Can you work these out from the model? Positions are in its coordinate system, mm. A direction names the side the tool comes from. Coordinates: 2 decimals unless noted, no trailing zeros. Order: outer loops, then holes, each group sorted by start corner. A loop starts at its lowest first (then second) coordinate and runs counter-clockwise, first axis right, second up.
Solid Edge part; units mm, degrees
sketch "Sketch1" plane through (0, 0, 0) normal (0, 0, 1) x (1, 0, 0)
  line L0 (-109.6195, 79.4537) -> (-109.6195, -60.5463)
  line L1 (-109.6195, -60.5463) -> (-99.6195, -70.5463)
  line L2 (-99.6195, -70.5463) -> (100.3805, -70.5463)
  line L3 (100.3805, -70.5463) -> (110.3805, -60.5463)
  line L4 (110.3805, -60.5463) -> (110.3805, 79.4537)
  line L5 (110.3805, 79.4537) -> (100.3805, 89.4537)
  line L6 (100.3805, 89.4537) -> (50.3805, 89.4537)
  line L7 (50.3805, 89.4537) -> (20.3805, 59.4537)
  line L8 (20.3805, 59.4537) -> (-19.6195, 59.4537)
  line L9 (-19.6195, 59.4537) -> (-49.6195, 89.4537)
  line L10 (-49.6195, 89.4537) -> (-99.6195, 89.4537)
  line L11 (-99.6195, 89.4537) -> (-109.6195, 79.4537)
  dimension "D1" = 110.3805
  dimension "D2" = 49.6195
extrude "Outside_ThinWallOptions" add sketch "Sketch1" along normal blind 50
shell "Inside" thickness 5 removed faces 1 at (-75.1528, -42.2796, 50)
sketch "Sketch2" plane through (0, 0, 0) normal (1, 0, 0) x (0, 1, 0)
  line L0 (84.4537, 25) -> (69.4537, 25)
  line L1 (69.4537, 25) -> (69.4537, 50)
  line L2 (69.4537, 50) -> (84.4537, 50)
  line L3 (84.4537, 50) -> (84.4537, 25)
  dimension "D1" = 84.4537
  dimension "D2" = 69.4537
extrude "Protrusion1" add sketch "Sketch2" against normal up to next and the other way up to next
1. I'm going to push flat-ended pins straight in: pin 1 (3 mm diameter, centred on x = -69, y = 45.5, fed in from +Z); pin 2 (16.5 mm diameter, centred on x = 10.5, y = 74.5, fed in from -Z); pin 3 (12.5 mm diameter, centred on x = -3, z = 43, fed in from +Y). Where does each tip first touch, or does it pass through?
Completed:
pin 1: stops at z = 5
pin 2: stops at z = 25
pin 3: stops at y = 84.45
2. Imagine slicing it at D-D on z = 31.5. Please give me the cut outline in (x, y).
Completed:
outline: (-109.62, -60.55) - (-99.62, -70.55) - (100.38, -70.55) - (110.38, -60.55) - (110.38, 79.45) - (100.38, 89.45) - (50.38, 89.45) - (45.38, 84.45) - (-44.62, 84.45) - (-49.62, 89.45) - (-99.62, 89.45) - (-109.62, 79.45) - close; hole (-104.62, -58.48) - (-97.55, -65.55) - (98.31, -65.55) - (105.38, -58.48) - (105.38, 77.38) - (98.31, 84.45) - (52.45, 84.45) - (22.45, 54.45) - (-21.69, 54.45) - (-51.69, 84.45) - (-97.55, 84.45) - (-104.62, 77.38) - close; hole (-29.62, 69.45) - (-19.62, 59.45) - (20.38, 59.45) - (30.38, 69.45) - close
3. Thinking about a two-plate mould opening in Y: for faces 1 (the flat face through (-104.55, 84.524, 24.65)), 2 (the flat face through (-104.69, -65.476, 24.65)), 3 (the flat face through (-104.62, 10, 27)), which applies, pulls with the +Y half, pulls with the -Y half, needs draft (parallel to the pull), parting line crosses it, or undercut?
Completed:
face 1: pulls with the +Y half
face 2: pulls with the -Y half
face 3: undercut
4. Imagine slicing it at B-B on y = 65.5. Please give me the cut outline in (x, z).
Completed:
outline: (-109.62, 0) - (-25.67, 0) - (-25.67, 50) - (-32.74, 50) - (-32.74, 5) - (-104.62, 5) - (-104.62, 50) - (-109.62, 50) - close; (26.43, 0) - (110.38, 0) - (110.38, 50) - (105.38, 50) - (105.38, 5) - (33.5, 5) - (33.5, 50) - (26.43, 50) - close
5. On a 3-axis mill with a long thin cutter (end or side, diameter ignored), from which of +Z, -Z, +X, -X, +Y, -Y can I reach the whole of each face in a straight line? I mean faces 4 (the flat face through (76, 89.454, 25)), 5 (the flat face through (1, 84.454, 38)), 6 (the flat face through (1, 69.454, 37)), 7 (the flat face through (105.38, 9, 27)). Say none if no direction works.
Completed:
face 4: +Z, -Z, +X, -X, +Y
face 5: +Z, -Z, +Y
face 6: +Z, -Z
face 7: +Z
6. Imagine slicing it at A-A on z = 19.5. Please give me the cut outline in (x, y), then the cut area to 3 significant figures.
Completed:
outline: (-109.62, -60.55) - (-99.62, -70.55) - (100.38, -70.55) - (110.38, -60.55) - (110.38, 79.45) - (100.38, 89.45) - (50.38, 89.45) - (20.38, 59.45) - (-19.62, 59.45) - (-49.62, 89.45) - (-99.62, 89.45) - (-109.62, 79.45) - close; hole (-104.62, -58.48) - (-97.55, -65.55) - (98.31, -65.55) - (105.38, -58.48) - (105.38, 77.38) - (98.31, 84.45) - (52.45, 84.45) - (22.45, 54.45) - (-21.69, 54.45) - (-51.69, 84.45) - (-97.55, 84.45) - (-104.62, 77.38) - close
area: 3,720 mm2
7. Imagine slicing it at C-C on x = 26. Please give me the cut outline in (y, z), then the cut area to 3 significant figures.
Completed:
outline: (-70.55, 0) - (65.07, 0) - (65.07, 50) - (58, 50) - (58, 5) - (-65.55, 5) - (-65.55, 50) - (-70.55, 50) - close; (69.45, 25) - (84.45, 25) - (84.45, 50) - (69.45, 50) - close
area: 1,600 mm2
8. Please list where these lines run through material, in increasing order: probe 1 along Y at (x, z) = (-75.5, 45); probe 2 along X at (y, z) = (46, 20.5); probe 3 along Y at (x, z) = (-17.5, 19).
Completed:
probe 1: y = -70.55 to -65.55, 84.45 to 89.45
probe 2: x = -109.62 to -104.62, 105.38 to 110.38
probe 3: y = -70.55 to -65.55, 54.45 to 59.45
